For this review, take the finished solid that the model builds, in its own axes (mm). Face numbers are marked on the shaded views. A direction names the side the tool comes from. Round coordinates to 2 decimals unless told otherwise and drop trailing zeros. Loops run counter-clockwise (first coordinate to the right, second up) from the corner with the lowest first, then second, coordinate; pieces in that order, holes last.
1) Take a section at A-A (x = 18). State the section outline as (y, z) points, then the cut area to 3 significant figures.
2) Wall thickness on L1, parallel to X at y = -1, z = 4.45; L2, parallel to Y at x = 5, z = 1.95; L3, parallel to Y at x = 7, z = 3.6: over which ranges is each line inside the solid? List them lowest first.
3) Take a section at C-C (x = -7). State the section outline as (y, z) points, then the cut area to 3 significant figures.
4) Take a section at B-B (z = 2.3). Give the number of separate pieces and of enclosed holes in the cut face, then the cut area to 3 significant figures.
5) Mouldability with a two-part tool opening along X and no side actions: class the marked faces 1, 2 and 3 as pulls with the +X half, pulls with the -X half, needs draft (parallel to the pull), parting line crosses it, or undercut.
6) Take a section at D-D (x = 1). State the section outline as (y, z) points.
7) Insertion check: pin 1 (10 mm diameter, centred on x = -3.5, y = 23, fed in from -Z); pin 2 (3 mm diameter, centred on x = -3.5, z = 2.5, fed in from -Y); pin 3 (3 mm diameter, centred on x = -4.5, z = 1, fed in from +Y). Each pin has a flat end and moves straight along its axis. Give the tip position at first contact, or say it passes through.
8) Tool access review of the marked faces 4 and 5: name each direction out of +Z, -Z, +X, -X, +Y, -Y from which nothing blocks a thin tool from reaching the whole face with its end or side.
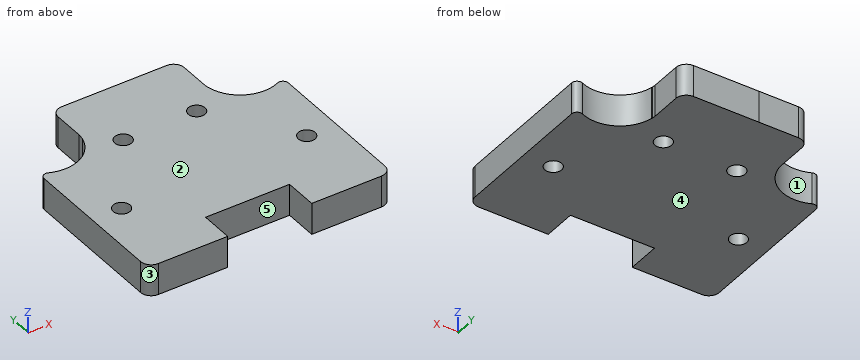
Autodesk Inventor part; units mm, degrees
ref_plane "Work Plane1" through (-23.2654, -35.3247, 0) normal (0, 0, 1) x (1, 0.0012, 0)
ref_plane "YZ Plane" through (0, 0, 0) normal (1, 0, 0) x (0, 1, 0)
ref_plane "XZ Plane" through (0, 0, 0) normal (0, 1, 0) x (-1, 0, 0)
sketch "Sketch1" plane through (0, 0, 0) normal (0, 0, 1) x (1, 0, 0)
  line L0 (-23.2294, -5.2752) -> (-23.2294, 25.7248)
  arc A0 (-23.2294, 25.7248) -> (-11.9794, 30.7248) centre (-18.9581, 31.2706) ccw
  line L1 (0.0206, 30.7248) -> (-11.9794, 30.7248)
  line L2 (0.0206, 30.7248) -> (12.0206, 30.7248)
  arc A1 (12.0206, 30.7248) -> (23.2706, 25.7248) centre (18.9993, 31.2706) ccw
  line L3 (23.2706, -5.2752) -> (23.2706, 25.7248)
  circle A2 centre (17.6456, 10.4258) radius 1.6
  circle A3 centre (-17.6044, 10.4258) radius 1.6
  line L4 (-23.2294, -5.2752) -> (23.2706, -5.2752)
  point P0 (0, 0)
  point P1 (0, -3.0755)
extrude "Extrusion1" add sketch "Sketch1" along normal blind 6
sketch "Sketch2" plane through (0, 0, 6) normal (0, 0, 1) x (1, 0, 0)
  circle A0 centre (-6.9972, 25.6961) radius 1.6
  circle A1 centre (7.0028, 25.7124) radius 1.6
  point P0 (0, 0)
extrude "Extrusion2" cut sketch "Sketch2" against normal through all
fillet "Fillet1" radius 1 4 edges at (-11.9794, 30.7248, 3) (-23.2294, 25.7248, 3) (12.0206, 30.7248, 3) (23.2706, 25.7248, 3)
fillet "Fillet2" radius 2 2 edges at (-23.2294, -5.2752, 3) (23.2706, -5.2752, 3)
sketch "Sketch3" plane through (0, 0, 6) normal (0, 0, 1) x (1, 0, 0)
  line L0 (0, 0.9807) -> (-8, 0.9807)
  line L1 (0, 0.9807) -> (8, 0.9807) construction
  line L2 (-8, 0.9807) -> (8, 0.9807)
  line L3 (8, 0.9807) -> (8, -5.2752)
  line L4 (21.2706, -5.2752) -> (-21.2294, -5.2752)
  line L5 (-8, 0.9807) -> (-8, -5.2752)
  point P0 (0, 0)
  dimension "d6" = 8
  dimension "d7" = 180
  dimension "d8" = 16
  dimension "d9" = 0
extrude "Extrusion3" cut sketch "Sketch3" against normal blind 10
sketch "Sketch4" plane through (0, 0, 6) normal (0, 0, 1) x (1, 0, 0)
  arc A0 (6.0143, -33.637) -> (7.9856, -35.2865) centre (7.9833, -33.2865) ccw
  line L0 (7.9856, -35.2865) -> (21.3237, -35.271)
  arc A1 (21.3237, -35.271) -> (23.3214, -33.2687) centre (21.3214, -33.271) ccw
  line L1 (23.3214, -33.2687) -> (23.2549, 23.9765)
  arc A2 (23.2549, 23.9765) -> (21.8449, 24.8874) centre (22.2549, 23.9753) ccw
  arc A3 (11.997, 30.7182) -> (21.8449, 24.8874) centre (18.9751, 31.2721) ccw
  line L2 (11.997, 30.7182) -> (11.9902, 36.6182)
  arc A4 (11.9902, 36.6182) -> (9.9879, 38.6159) centre (9.9902, 36.6159) ccw
  line L3 (9.9879, 38.6159) -> (2.4879, 38.6072)
  arc A5 (2.4879, 38.6072) -> (1.489, 37.606) centre (2.489, 37.6072) ccw
  line L4 (1.489, 37.606) -> (1.4937, 33.606)
  line L5 (1.4937, 33.606) -> (2.7437, 33.6075)
  line L6 (2.7437, 33.6075) -> (2.747, 30.7075)
  line L7 (2.747, 30.7075) -> (1.547, 30.7061)
  line L8 (1.547, 30.7061) -> (1.5587, 20.7061)
  line L9 (1.5587, 20.7061) -> (10.0087, 20.7159)
  arc A6 (12.011, 18.7182) -> (10.0087, 20.7159) centre (10.011, 18.7159) ccw
  line L10 (12.011, 18.7182) -> (12.0365, -3.2818)
  arc A7 (12.0365, -3.2818) -> (14.0389, -5.2794) centre (14.0365, -3.2794) ccw
  line L11 (14.0389, -5.2794) -> (16.2889, -5.2768)
  arc A8 (18.2912, -7.2745) -> (16.2889, -5.2768) centre (16.2912, -7.2768) ccw
  line L12 (18.2912, -7.2745) -> (18.3109, -24.2745)
  arc A9 (16.3133, -26.2768) -> (18.3109, -24.2745) centre (16.3109, -24.2768) ccw
  line L13 (16.3133, -26.2768) -> (-16.1867, -26.3146)
  arc A10 (-18.189, -24.3169) -> (-16.1867, -26.3146) centre (-16.189, -24.3146) ccw
  line L14 (-18.189, -24.3169) -> (-18.2088, -7.3169)
  arc A11 (-16.2111, -5.3146) -> (-18.2088, -7.3169) centre (-16.2088, -7.3146) ccw
  line L15 (-16.2111, -5.3146) -> (-13.9611, -5.312)
  arc A12 (-13.9611, -5.312) -> (-11.9634, -3.3096) centre (-13.9634, -3.312) ccw
  line L16 (-11.9634, -3.3096) -> (-11.989, 18.6903)
  arc A13 (-9.9913, 20.6927) -> (-11.989, 18.6903) centre (-9.989, 18.6927) ccw
  line L17 (-9.9913, 20.6927) -> (-1.5413, 20.7025)
  line L18 (-1.5413, 20.7025) -> (-1.553, 30.7025)
  line L19 (-1.553, 30.7025) -> (-2.753, 30.7011)
  line L20 (-2.753, 30.7011) -> (-2.7563, 33.6011)
  line L21 (-2.7563, 33.6011) -> (-1.5063, 33.6025)
  line L22 (-1.5063, 33.6025) -> (-1.511, 37.6025)
  arc A14 (-1.511, 37.6025) -> (-2.5121, 38.6014) centre (-2.511, 37.6014) ccw
  line L23 (-2.5121, 38.6014) -> (-10.0121, 38.5926)
  arc A15 (-10.0121, 38.5926) -> (-12.0098, 36.5903) centre (-10.0098, 36.5926) ccw
  line L24 (-12.0098, 36.5903) -> (-12.0029, 30.6903)
  arc A16 (-21.8372, 24.8367) -> (-12.0029, 30.6903) centre (-18.9823, 31.228) ccw
  arc A17 (-21.8372, 24.8367) -> (-23.2451, 23.9225) centre (-22.2451, 23.9236) ccw
  line L25 (-23.2451, 23.9225) -> (-23.1786, -33.3227)
  arc A18 (-23.1786, -33.3227) -> (-21.1762, -35.3204) centre (-21.1786, -33.3204) ccw
  line L26 (-21.1762, -35.3204) -> (-7.8381, -35.3049)
  arc A19 (-7.8381, -35.3049) -> (-5.8706, -33.6509) centre (-7.8405, -33.3049) ccw
  arc A20 (6.0143, -33.637) -> (-5.8706, -33.6509) centre (0.073, -34.6948) ccw
  circle A21 centre (17.6456, 10.4258) radius 1.6
  circle A22 centre (-17.6044, 10.3848) radius 1.6
  circle A23 centre (7.0029, 25.7124) radius 1.6
  circle A24 centre (-6.9971, 25.6961) radius 1.6
  line L27 (11.1501, 30.7248) -> (-11.1088, 30.7248)
  line L28 (-2.5121, 38.6014) -> (2.4879, 38.6072)
  line L29 (-12.1907, 29.5326) -> (12.1947, 29.5326)
  point P0 (0, 0)
ref_plane "Work Plane1" through (-23.2654, -35.3247, 0) normal (0, 0, 1) x (1, 0.0012, 0)
extrude "Extrusion4" add sketch "Sketch4" against normal up to surface (6 mm away) contours L29 L8 L7 L6 L5 L4 A5 L3 A4 L2 A3 | L29 L18 L19 L20 L27 L6 L7 L8 | A16 L24 A15 L23 A14 L22 L21 L20 L19 L18 L29 | A5 L4 L5 L6 L27 L20 L21 L22 A14 L28
properties part number "Hotend Slide Part3" material "PET Plastic"
Response:
1. outline: (-5.28, 0) - (8.87, 0) - (8.87, 6) - (-5.28, 6) - close; (11.99, 0) - (24.34, 0) - (24.34, 6) - (11.99, 6) - close
1. area: 159 mm2
2. L1: x = -23.23 to -8, 8 to 23.27
2. L2: y = 0.98 to 38.61
2. L3: y = 0.98 to 24.11, 27.31 to 38.61
3. outline: (0.98, 0) - (24.1, 0) - (24.1, 6) - (0.98, 6) - close; (27.3, 0) - (38.6, 0) - (38.6, 6) - (27.3, 6) - close
3. area: 206 mm2
4. separate pieces: 1
4. enclosed holes: 4
4. area: 1,610 mm2
5. face 1: undercut
5. face 2: needs draft
5. face 3: pulls with the -X half
6. outline: (0.98, 0) - (38.61, 0) - (38.61, 6) - (0.98, 6) - close
7. pin 1: stops at z = 0
7. pin 2: stops at y = 0.98
7. pin 3: stops at y = 38.6
8. face 4: -Z, +X, -X, +Y, -Y
8. face 5: +Z, -Z, -Y
